```python
from build123d import *

# Parameters (mm, degrees)
SKETCH1_R           = 1
BOSS_EXTRUDE1_DEPTH = 0.2


with BuildPart() as part:
    # Sketch1 → Boss-Extrude1 (new body)
    with BuildSketch(Plane.XY):
        with BuildLine():
            Line((-0.238423982, 1.985737648), (-0.766818617, 6.386524482))
            ThreePointArc((-0.766818617, 6.386524482), (-0.773753956, 6.48594667), (-0.77075837, 6.585565427))
            Line((-0.77075837, 6.585565427), (-0.303191424, 12.423982653))
            ThreePointArc((-0.303191424, 12.423982653), (-0.300798174, 12.463865246), (-0.3, 12.503811607))
            Line((-0.3, 12.503811607), (-0.3, 13.862922443))
            ThreePointArc((-0.3, 13.862922443), (-2.008962857, 15.057847822), (-2.020381908, 17.143098483))
            ThreePointArc((-2.020381908, 17.143098483), (-0.856036284, 18.990797554), (0, 21))
            ThreePointArc((0, 21), (0.856036284, 18.990797554), (2.020381908, 17.143098483))
            ThreePointArc((2.020381908, 17.143098483), (2.008962857, 15.057847822), (0.3, 13.862922443))
            Line((0.3, 13.862922443), (0.3, 12.503811607))
            ThreePointArc((0.3, 12.503811607), (0.300798174, 12.463865246), (0.303191424, 12.423982653))
            Line((0.303191424, 12.423982653), (0.77075837, 6.585565427))
            ThreePointArc((0.77075837, 6.585565427), (0.773753956, 6.48594667), (0.766818617, 6.386524482))
            Line((0.766818617, 6.386524482), (0.238423982, 1.985737648))
            ThreePointArc((0.238423982, 1.985737648), (0, -2), (-0.238423982, 1.985737648))
        make_face()
        Circle(SKETCH1_R, mode=Mode.SUBTRACT)
    extrude(amount=BOSS_EXTRUDE1_DEPTH)


solid = part.part
```
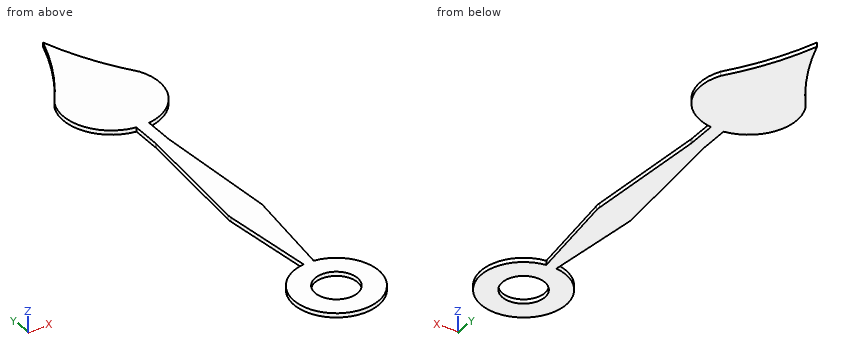
Geometry: final body of the model. Coordinates: model frame, mm. Coordinates: 2 decimals unless noted, no trailing zeros. Order: outer loops, then holes, each group sorted by start corner. A loop starts at its lowest first (then second) coordinate and runs counter-clockwise, first axis right, second up. Notation, with made-up numbers: (80.25, 52) - (123.25, 52) arc R22 cw to (123.25, 58) - close; hole circle Ø8 at (-18.5, 6). An arc over 180 degrees is marked (long way). Write each question's results on one line, items separated by ' | '.
1) Section C-C, the plane x = -1.5. Return loops of the section in (y, z), plus the area to 3 significant figures.
Results list:
outline: (-1.32, 0) - (1.32, 0) - (1.32, 0.2) - (-1.32, 0.2) - close; (14.41, 0) - (17.89, 0) - (17.89, 0.2) - (14.41, 0.2) - close | area: 1.23 mm^2
2) Section A-A, the plane z = 0.15. Return loops of the section in (x, y).
Results list:
outline: (-2.02, 17.14) arc R2.27 ccw to (-0.3, 13.86) - (-0.3, 12.5) arc R1 cw to (-0.3, 12.42) - (-0.77, 6.59) arc R1 ccw to (-0.77, 6.39) - (-0.24, 1.99) arc R2 ccw (long way) to (0.24, 1.99) - (0.77, 6.39) arc R1 ccw to (0.77, 6.59) - (0.3, 12.42) arc R1 cw to (0.3, 12.5) - (0.3, 13.86) arc R2.27 ccw to (2.02, 17.14) arc R13.7 cw to (0, 21) arc R13.7 cw to start; hole circle Ø2 at (0, 0)
3) Section B-B, the plane y = 0. Return loops of the section in (x, z).
Results list:
outline: (-2, 0) - (-1, 0) - (-1, 0.2) - (-2, 0.2) - close; (1, 0) - (2, 0) - (2, 0.2) - (1, 0.2) - close
4) Line query: line 1 (Y direction, x = -1.75, z = 0.1); line 2 (X direction, y = 11.75, z = 0.1); line 3 (X direction, y = 8, z = 0.1). Output: solid intervals per line, ascending. Write a range as from..to.
Results list:
line 1: -0.97..0.97, 14.67..17.52 | line 2: -0.36..0.36 | line 3: -0.66..0.66
5) Section D-D, the plane y = 8. Return loops of the section in (x, z), plus the area to 3 significant figures.
Results list:
outline: (-0.66, 0) - (0.66, 0) - (0.66, 0.2) - (-0.66, 0.2) - close | area: 0.263 mm^2
